Check sheet for the modelled part. Datum: model origin and axes. Units: mm. Face numbers are marked on the shaded views. A direction names the side the tool comes from. Give positions to 0.01 mm unless a question says otherwise; leave off trailing zeros. Order: outer loops, then holes, each group sorted by start corner. A loop starts at its lowest first (then second) coordinate and runs counter-clockwise, first axis right, second up.
```python
from build123d import *

# Parameters (mm, degrees)
F1_DEPTH = 5.08
F0_W     = 129.5400008702
F0_H     = 5.08
F2_DEPTH = 55.88
F4_DEPTH = 5.08
F6_START = 30.48
F6_DEPTH = 5.08
F7_START = -25.4
F7_DEPTH = 5.08


# Not quite as in the source:
# - a feature names something its author has since deleted; it is built from what else it names


with BuildPart() as f1:
    # F0 (on Front) → F1 (new body)
    with BuildSketch(Plane.XZ):
        with BuildLine():
            Line((-62.1654726565, 25.9080137503), (-62.1654726565, -33.7819862497))
            Line((-62.1654726565, -33.7819862497), (67.3745282138, -33.7819862497))
            Line((67.3745282138, -33.7819862497), (67.3745282138, 25.9080137503))
            ThreePointArc((67.3745282138, 25.9080137503), (58.4845213386, 34.7980137503), (49.5945282137, 25.908))
            Line((49.5945282137, 25.908), (49.5945282137, 6.35))
            ThreePointArc((49.5945282137, 6.35), (47.7346562743, 1.8598719395), (43.2445282137, 0))
            Line((43.2445282137, 0), (-38.0354726565, 0))
            ThreePointArc((-38.0354726565, 0), (-42.525600717, 1.8598719395), (-44.3854726565, 6.35))
            Line((-44.3854726565, 6.35), (-44.3854726565, 25.908))
            ThreePointArc((-44.3854726565, 25.908), (-53.2754657813, 34.7980137503), (-62.1654726565, 25.9080137503))
        make_face()
        with BuildLine():
            ThreePointArc((-56.4504726565, 25.9080137503), (-53.2754726565, 29.0830137503), (-50.1004726565, 25.9080137503))
            Line((-50.1004726565, 25.9080137503), (-50.1004726565, -24.8919862497))
            ThreePointArc((-50.1004726565, -24.8919862497), (-53.2754726565, -28.0669862497), (-56.4504726565, -24.8919862497))
            Line((-56.4504726565, -24.8919862497), (-56.4504726565, 25.9080137503))
        make_face(mode=Mode.SUBTRACT)
        with BuildLine():
            ThreePointArc((55.3095273435, 25.9080137503), (58.4845273435, 29.0830137503), (61.6595273435, 25.9080137503))
            Line((61.6595273435, 25.9080137503), (61.6595273435, -24.8919862497))
            ThreePointArc((61.6595273435, -24.8919862497), (58.4845273435, -28.0669862497), (55.3095273435, -24.8919862497))
            Line((55.3095273435, -24.8919862497), (55.3095273435, 25.9080137503))
        make_face(mode=Mode.SUBTRACT)
    extrude(amount=F1_DEPTH)

    # F0 (on Front) → F2 (join)
    with BuildSketch(Plane.XZ):
        with Locations((2.6045277786, -36.3219862497)):
            Rectangle(F0_W, F0_H)
    extrude(amount=F2_DEPTH)

    # F3 (on face) → F4 (cut)
    with BuildSketch(Plane.XY.offset(-33.7819862497)):
        with BuildLine():
            ThreePointArc((-53.2754726565, -55.88), (-59.5616519412, -53.2761792847), (-62.1654726565, -46.99))
            Line((-62.1654726565, -46.99), (-62.1654726565, -55.88))
            Line((-62.1654726565, -55.88), (-53.2754726565, -55.88))
        make_face()
        with BuildLine():
            ThreePointArc((67.3745282138, -46.99), (64.7707071908, -53.2761795924), (58.4845273435, -55.88))
            Line((58.4845273435, -55.88), (67.3745282138, -55.88))
            Line((67.3745282138, -55.88), (67.3745282138, -46.99))
        make_face()
    extrude(amount=-F4_DEPTH, mode=Mode.SUBTRACT)

    # F5 (on Right) → F6 (join)
    with BuildSketch(Plane.YZ.offset(F6_START)):
        Polygon((-5.08, -33.7819862497), (-5.08, -8.3819862497), (-30.48, -33.7819862497), align=None)
    extrude(amount=F6_DEPTH)

    # F5 (on Right) → F7 (join)
    with BuildSketch(Plane.YZ.offset(F7_START)):
        Polygon((-5.08, -33.7819862497), (-5.08, -8.3819862497), (-30.48, -33.7819862497), align=None)
    extrude(amount=-F7_DEPTH)


solid = f1.part
```
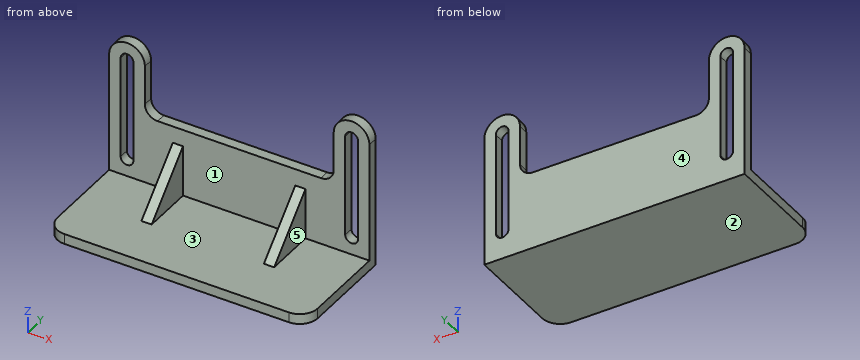
(1) Release check for a two-part mould opening along X. For the marked faces 3, 4 and 5 record: released by +X, released by -X, zero draft, split by the parting line, or undercut.
(2) Sectioned sample at B-B (z = -20). Enter the section's corners in (x, y), plus the area to 3 significant figures.
(3) Sectioned sample at D-D (y = -10.5). Enter the section's corners in (x, z).
(4) Sectioned sample at A-A (z = 9). Enter the section's corners in (x, y), plus the area to 3 significant figures.
(5) Tool access check on the marked faces 1 and 2. Record the directions out of +Z, -Z, +X, -X, +Y, -Y that give a thin tool (end or side, any length) a straight path to the whole face; none if there is none.
(6) Go/stop test with flat-tipped pins: P1, Ø2, axis at y = -9, z = -27.5, coming from the +X side; P2, Ø2, axis at x = 5, y = -31.5, coming from the +Z side; P3, Ø20.5, axis at y = -15.5, z = -23.5, coming from the -X side; P4, Ø1.5, axis at x = -14, z = 1.5, coming from the +Y side. Record where each tip stops, or that it passes through.
(7) Thickness scan on L1, parallel to X at y = -4.5, z = -13; L2, parallel to X at y = -16.5, z = -25; L3, parallel to Y at x = -3, z = -21.5. Record the ranges inside material, lowest first.
(8) Sectioned sample at C-C (x = 1.5). Enter the section's corners in (y, z), plus the area to 3 significant figures.
Values follow:
1. face 3: undercut
1. face 4: zero draft
1. face 5: released by +X
2. outline: (-62.17, -5.08) - (-56.45, -5.08) - (-56.45, 0) - (-62.17, 0) - close; (-50.1, -5.08) - (-30.48, -5.08) - (-30.48, -16.7) - (-25.4, -16.7) - (-25.4, -5.08) - (30.48, -5.08) - (30.48, -16.7) - (35.56, -16.7) - (35.56, -5.08) - (55.31, -5.08) - (55.31, 0) - (-50.1, 0) - close; (61.66, -5.08) - (67.37, -5.08) - (67.37, 0) - (61.66, 0) - close
2. area: 712 mm2
3. outline: (-62.17, -38.86) - (67.37, -38.86) - (67.37, -33.78) - (35.56, -33.78) - (35.56, -13.8) - (30.48, -13.8) - (30.48, -33.78) - (-25.4, -33.78) - (-25.4, -13.8) - (-30.48, -13.8) - (-30.48, -33.78) - (-62.17, -33.78) - close
4. outline: (-62.17, -5.08) - (-56.45, -5.08) - (-56.45, 0) - (-62.17, 0) - close; (-50.1, -5.08) - (-44.39, -5.08) - (-44.39, 0) - (-50.1, 0) - close; (49.59, -5.08) - (55.31, -5.08) - (55.31, 0) - (49.59, 0) - close; (61.66, -5.08) - (67.37, -5.08) - (67.37, 0) - (61.66, 0) - close
4. area: 116 mm2
5. face 1: +Z, -Y
5. face 2: -Z, +X, -X, +Y, -Y
6. P1: stops at x = 35.56
6. P2: stops at z = -33.78
6. P3: stops at x = -30.48
6. P4: passes through
7. L1: x = -62.17 to -56.45, -50.1 to 55.31, 61.66 to 67.37
7. L2: x = -30.48 to -25.4, 30.48 to 35.56
7. L3: y = -5.08 to 0
8. outline: (-55.88, -38.86) - (0, -38.86) - (0, 0) - (-5.08, 0) - (-5.08, -33.78) - (-55.88, -33.78) - close
8. area: 455 mm2
